```python
from build123d import *

# Parameters (mm, degrees)
SKETCH1_W           = 35
SKETCH1_H           = 85
BOSS_EXTRUDE1_DEPTH = 10
SKETCH2_W           = 31
SKETCH2_H           = 81
CUT_EXTRUDE1_DEPTH  = 8
SKETCH3_W           = 9
SKETCH3_H           = 9
SKETCH3_R           = 1.25
BOSS_EXTRUDE2_DEPTH = 8
CUT_EXTRUDE3_START  = -10
SKETCH4_R           = 1.25
CUT_EXTRUDE3_DEPTH  = 10
SKETCH5_R           = 3
CUT_EXTRUDE4_DEPTH  = 5
FILLET1_R           = 1
SKETCH6_R           = 2.5
CUT_EXTRUDE5_DEPTH  = 5


with BuildPart() as part:
    # Sketch1 → Boss-Extrude1 (new body)
    with BuildSketch(Plane(origin=(0, 0, 0), x_dir=(1, 0, 0), z_dir=(0, 1, 0))):
        Rectangle(SKETCH1_W, SKETCH1_H)
    extrude(amount=BOSS_EXTRUDE1_DEPTH)

    # Sketch2 → Cut-Extrude1 (cut)
    with BuildSketch(Plane.XZ):
        Rectangle(SKETCH2_W, SKETCH2_H)
    extrude(amount=-CUT_EXTRUDE1_DEPTH, mode=Mode.SUBTRACT)

    # Sketch3 → Boss-Extrude2 (add)
    # profile 1 of 3: a face of its own
    with BuildSketch(Plane.XZ.offset(-8)):
        with Locations((-11, 36)):
            Rectangle(SKETCH3_W, SKETCH3_H)
        with Locations(Location((-11, 36, 0), (0, 0, 270))):
            Circle(SKETCH3_R, mode=Mode.SUBTRACT)
    # profile 2 of 3: a face of its own
    with BuildSketch(Plane.XZ.offset(-8)):
        with Locations((11, 36)):
            Rectangle(SKETCH3_W, SKETCH3_H)
        with Locations(Location((11, 36, 0), (0, 0, 270))):
            Circle(SKETCH3_R, mode=Mode.SUBTRACT)
    # profile 3 of 3: a face of its own
    with BuildSketch(Plane.XZ.offset(-8)):
        with Locations((11, -36)):
            Rectangle(SKETCH3_W, SKETCH3_H)
        with Locations(Location((11, -36, 0), (0, 0, 270))):
            Circle(SKETCH3_R, mode=Mode.SUBTRACT)
    extrude(amount=BOSS_EXTRUDE2_DEPTH)

    # Sketch4 → Cut-Extrude3 (cut)
    with BuildSketch(Plane.XZ.offset(CUT_EXTRUDE3_START)):
        with Locations(Location((-11, 36, 0), (0, 0, 270))):
            Circle(SKETCH4_R)
        with Locations(Location((11, 36, 0), (0, 0, 270))):
            Circle(SKETCH4_R)
        with Locations(Location((11, -36, 0), (0, 0, 270))):
            Circle(SKETCH4_R)
    extrude(amount=CUT_EXTRUDE3_DEPTH, mode=Mode.SUBTRACT)

    # Sketch5 → Cut-Extrude4 (cut)
    with BuildSketch(Plane(origin=(0, 10, 0), x_dir=(1, 0, 0), z_dir=(0, 1, 0))):
        with Locations(Location((11, -36, 0), (0, 0, 270))):
            Circle(SKETCH5_R)
        with Locations(Location((-11, -36, 0), (0, 0, 270))):
            Circle(SKETCH5_R)
        with Locations(Location((11, 36, 0), (0, 0, 270))):
            Circle(SKETCH5_R)
    extrude(amount=-CUT_EXTRUDE4_DEPTH, mode=Mode.SUBTRACT)

    # Fillet1
    fillet1_edges = [part.edges().sort_by_distance(p)[0] for p in [
        (-17.5, 10, 0),
        (0, 10, 42.5),
    ]]
    fillet(fillet1_edges, radius=FILLET1_R)

    # Sketch6 → Cut-Extrude5 (cut)
    with BuildSketch(Plane(origin=(0, 10, 0), x_dir=(1, 0, 0), z_dir=(0, 1, 0))):
        with Locations(Location((2.5, -3.5, 0), (0, 0, 270))):
            Circle(SKETCH6_R)
    extrude(amount=-CUT_EXTRUDE5_DEPTH, mode=Mode.SUBTRACT)


solid = part.part
```
The listing builds one solid part. Answer for the finished solid, in the listing's coordinates (mm). A direction names the side the tool comes from. Coordinates: 2 decimals unless noted, no trailing zeros. Order: outer loops, then holes, each group sorted by start corner. A loop starts at its lowest first (then second) coordinate and runs counter-clockwise, first axis right, second up. Notation, with made-up numbers: M -11.75,44 L 17.25,44 A18 ccw 17.25,55 Z; hole C 67.25,27 d6. An arc over 180 degrees is marked long. Answer as a JSON object with one key per item and string values. Group by question number.
1. Section A-A on z = 36 is taken. Write down the section's boundary in (x, y), then the cut area to 3 significant figures.
2. Determine the mould class of faces 4 (the cylindrical face through (12.24, 2.54, -35.84)), 5 (the flat face through (-16, 0, 3)), 6 (the flat face through (0, 5, -42.5)) for opening direction Z: released by +Z, released by -Z, zero draft, split by the parting line, or undercut.
3. Flat-ended cylindrical pins translate along their axes: P1, Ø15.5, axis at x = 7.5, z = -2.5, coming from the -Y side; P2, Ø1.8, axis at x = -11.5, z = 34.5, coming from the +Y side. Find the tip coordinate at first contact, or state that the pin passes through.
4. Section D-D on z = -36 is taken. Write down the section's boundary in (x, y).
5. A tool of negligible diameter and unlimited length cuts with its end or side. For faces 1 (the cylindrical face through (0.28, 9.01, 4.65)), 2 (the flat face through (10, 5, 37)), 3 (the flat face through (11, 4, -31.5)), from which of +Z, -Z, +X, -X, +Y, -Y can it reach the whole face along a straight path? Write none if from no direction.
6. Straight lines are drawn through the part: line 1 (X direction, y = 7.15, z = 36); line 2 (X direction, y = 8.55, z = 36); line 3 (X direction, y = 1.2, z = 36). For each, find the intervals that lie inside material, in ascending order.
7. Section B-B on x = 2.5 is taken. Write down the section's boundary in (y, z).
8. Section C-C on y = 1 is taken. Write down the section's boundary in (x, z), then the cut area to 3 significant figures.
Values follow:
{
 "1": {"outline": "M -17.5,0 L -12.25,0 L -12.25,5 L -14,5 L -14,10 L -16.5,10 A1 ccw -17.5,9 Z; M -9.75,0 L -6.5,0 L -6.5,8 L 6.5,8 L 6.5,0 L 9.75,0 L 9.75,5 L 8,5 L 8,10 L -8,10 L -8,5 L -9.75,5 Z; M 12.25,0 L 17.5,0 L 17.5,10 L 14,10 L 14,5 L 12.25,5 Z", "area": "161 mm2"},
 "2": {"face 4": "undercut", "face 5": "zero draft", "face 6": "released by -Z"},
 "3": {"P1": "y = 8", "P2": "y = 5"},
 "4": {"outline": "M -17.5,0 L -15.5,0 L -15.5,8 L 6.5,8 L 6.5,0 L 9.75,0 L 9.75,5 L 8,5 L 8,10 L -16.5,10 A1 ccw -17.5,9 Z; M 12.25,0 L 17.5,0 L 17.5,10 L 14,10 L 14,5 L 12.25,5 Z"},
 "5": {"face 1": "+Y, -Y", "face 2": "+Y", "face 3": "-Y"},
 "6": {"line 1": "-17.5 to -14, -8 to -6.5, 6.5 to 8, 14 to 17.5", "line 2": "-17.5 to -14, -8 to 8, 14 to 17.5", "line 3": "-17.5 to -12.25, -9.75 to -6.5, 6.5 to 9.75, 12.25 to 17.5"},
 "7": {"outline": "M 0,-42.5 L 10,-42.5 L 10,1 L 8,1 L 8,-40.5 L 0,-40.5 Z; M 0,40.5 L 8,40.5 L 8,6 L 10,6 L 10,41.5 A1 ccw 9,42.5 L 0,42.5 Z"},
 "8": {"outline": "M -17.5,-42.5 L 17.5,-42.5 L 17.5,42.5 L -17.5,42.5 Z; hole M -15.5,-40.5 L 6.5,-40.5 L 6.5,-31.5 L 15.5,-31.5 L 15.5,31.5 L 6.5,31.5 L 6.5,40.5 L -6.5,40.5 L -6.5,31.5 L -15.5,31.5 Z; hole C -11,36 d2.5; hole C 11,-36 d2.5; hole C 11,36 d2.5", "area": "692 mm2"}
}
